Geometry: final body of the model. Coordinates: model frame, mm. Face numbers are marked on the shaded views. A direction names the side the tool comes from. Round coordinates to 2 decimals unless told otherwise and drop trailing zeros. Write each loop counter-clockwise with the first axis right and the second up, starting at its lowest first coordinate (ties: lowest second). Pieces come first, ordered by that corner, then holes.
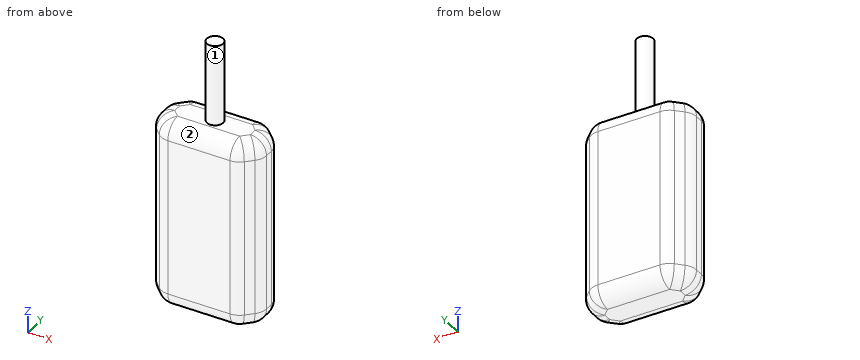
from build123d import *

# Parameters (mm, degrees)
SKETCH_1_W      = 20
SKETCH_1_H      = 10
EXTRUDE_1_DEPTH = 35
CHAMFER_2_SIZE  = 3
FILLET_1_R      = 3
SKETCH_2_R      = 1.5
EXTRUDE_2_DEPTH = 15


with BuildPart() as part:
    # 草图1 → 凸台-拉伸1 (new body)
    with BuildSketch(Plane.XY):
        with Locations((10, 5)):
            Rectangle(SKETCH_1_W, SKETCH_1_H)
    extrude(amount=EXTRUDE_1_DEPTH)

    # 倒角2
    chamfer_2_edges = [part.edges().sort_by_distance(p)[0] for p in [
        (0, 0, 17.5),
        (0, 10, 17.5),
        (20, 10, 17.5),
        (20, 0, 17.5),
    ]]
    chamfer(chamfer_2_edges, length=CHAMFER_2_SIZE)

    # 圆角1
    fillet_1_edges = [part.edges().sort_by_distance(p)[0] for p in [
        (20, 5, 0),
        (20, 5, 35),
        (20, 7, 17.5),
        (20, 3, 17.5),
        (10, 0, 0),
        (0, 5, 0),
        (10, 10, 0),
        (18.5, 8.5, 0),
        (1.5, 8.5, 0),
        (1.5, 1.5, 0),
        (18.5, 1.5, 0),
        (10, 0, 35),
        (3, 0, 17.5),
        (17, 0, 17.5),
        (10, 10, 35),
        (0, 5, 35),
        (18.5, 8.5, 35),
        (1.5, 8.5, 35),
        (1.5, 1.5, 35),
        (18.5, 1.5, 35),
        (0, 7, 17.5),
        (0, 3, 17.5),
        (17, 10, 17.5),
        (3, 10, 17.5),
    ]]
    fillet(fillet_1_edges, radius=FILLET_1_R)

    # 草图2 → 凸台-拉伸2 (add)
    with BuildSketch(Plane.XY.offset(35)):
        with Locations(Location((10, 5, 0), (0, 0, 180))):
            Circle(SKETCH_2_R)
    extrude(amount=EXTRUDE_2_DEPTH)


solid = part.part
1) Line query: probe 1 along Z at (x, y) = (4.5, 4.25); probe 2 along X at (y, z) = (6, 18.5); probe 3 along X at (y, z) = (4.5, 33). Output: solid intervals per line, ascending.
2) Section A-A on y = 5. Output: boundary loops of the cut face in (x, z).
3) Section B-B on x = 8. Output: boundary loops of the cut face in (y, z), plus the area to 3 significant figures.
4) Reachability of the marked faces 1 and 2 from +Z, -Z, +X, -X, +Y, -Y: full face, straight path, thin tool, end or side. Return the list, or none.
5) Section D-D on x = 10. Output: boundary loops of the cut face in (y, z).
6) Section C-C on z = 42. Output: boundary loops of the cut face in (x, y), plus the area to 3 significant figures.
7) First-contact query: P1, Ø1, axis at y = 2.5, z = 24.5, coming from the +X side; P2, Ø5, axis at x = 17.5, y = 1, coming from the -Z side; P3, Ø12, axis at x = 9.5, z = 16.5, coming from the -Y side; P4, Ø4, axis at y = 2.5, z = 42.5, coming from the -X side. Flat tips, straight axial feed; report the tip coordinate or a pass-through.
Filled in:
1. probe 1: z = 0 to 35
1. probe 2: x = 0.01 to 19.99
1. probe 3: x = 0.17 to 19.83
2. outline: (0, 3) arc R3 ccw to (3, 0) - (17, 0) arc R3 ccw to (20, 3) - (20, 32) arc R3 ccw to (17, 35) - (11.5, 35) - (11.5, 50) - (8.5, 50) - (8.5, 35) - (3, 35) arc R3 ccw to (0, 32) - close
3. outline: (0, 3) arc R3 ccw to (3, 0) - (7, 0) arc R3 ccw to (10, 3) - (10, 32) arc R3 ccw to (7, 35) - (3, 35) arc R3 ccw to (0, 32) - close
3. area: 342 mm2
4. face 1: +Z
4. face 2: +Z, +X, -X, -Y
5. outline: (0, 3) arc R3 ccw to (3, 0) - (7, 0) arc R3 ccw to (10, 3) - (10, 32) arc R3 ccw to (7, 35) - (6.5, 35) - (6.5, 50) - (3.5, 50) - (3.5, 35) - (3, 35) arc R3 ccw to (0, 32) - close
6. outline: circle Ø3 at (10, 5)
6. area: 7.07 mm2
7. P1: stops at x = 19.73
7. P2: stops at z = 0
7. P3: stops at y = 0
7. P4: stops at x = 8.59
